Design review of the part built by this model. Coordinates are the model's own, in mm. A direction names the side the tool comes from. Coordinates: 2 decimals unless noted, no trailing zeros. Order: outer loops, then holes, each group sorted by start corner. A loop starts at its lowest first (then second) coordinate and runs counter-clockwise, first axis right, second up. Notation, with made-up numbers: M 5.25,73.25 L 12.25,73.25 A23 ccw 12.25,110.25 Z; hole C 73,24.25 d3. An arc over 180 degrees is marked long. Answer in a Markdown table with one row per item.
from build123d import *

# Parameters (mm, degrees)
SKETCH1_R           = 4.7625
BOSS_EXTRUDE1_DEPTH = 65.1002
SKETCH2_W           = 9.525
SKETCH2_H           = 2.54
CUT_EXTRUDE1_DEPTH  = 3.175
CHAMFER1_SIZE       = 0.508


with BuildPart() as part:
    # Sketch1 → Boss-Extrude1 (new body)
    with BuildSketch(Plane.XY):
        Circle(SKETCH1_R)
    extrude(amount=BOSS_EXTRUDE1_DEPTH)

    # Sketch2 → Cut-Extrude1 (cut)
    with BuildSketch(Plane.XY.offset(65.1002)):
        Rectangle(SKETCH2_W, SKETCH2_H)
    extrude(amount=-CUT_EXTRUDE1_DEPTH, mode=Mode.SUBTRACT)

    # Chamfer1
    chamfer1_edges = [part.edges().sort_by_distance(p)[0] for p in [
        (0, 4.7625, 65.1002),
        (0, -4.7625, 65.1002),
    ]]
    chamfer(chamfer1_edges, length=CHAMFER1_SIZE)


solid = part.part
(1) Insertion check: pin 1 Ø5 at (x, z) = (3, 56.5) entering from +Y; pin 2 Ø0.8 at (x, y) = (1, 0.5) entering from +Z. Each pin has a flat end and moves straight along its axis. Give the tip position at first contact, or say it passes through.
Return value:
| item | result |
|---|---|
| pin 1 | stops at y = 4.74 |
| pin 2 | stops at z = 61.93 |
(2) Draft analysis for pull direction Y (two halves, no side actions). For faces 3 (the conical face through (-0.08, -4.391, 64.963)), 4 (the flat face through (0, 0, 0)), 5 (the flat face through (0, 1.27, 64)), 6 (the conical face through (0.08, 4.391, 64.963)), state which applies: pulls with the +Y half, pulls with the -Y half, needs draft (parallel to the pull), parting line crosses it, or undercut.
Return value:
| item | result |
|---|---|
| face 3 | pulls with the -Y half |
| face 4 | needs draft |
| face 5 | undercut |
| face 6 | pulls with the +Y half |
(3) For line 1 along X through (y, z) = (-2.5, 52.5); line 2 along Z through (x, y) = (-2.75, -1); line 3 along X through (y, z) = (1.25, 17.5), list the stretches that pass through material, from the lowest coordinate up. Write a range as from..to.
Return value:
| item | result |
|---|---|
| line 1 | x = -4.05..4.05 |
| line 2 | z = 0..61.93 |
| line 3 | x = -4.6..4.6 |
(4) Add section A-A, the plane y = 0. Give the boundary of the cut face in (x, z).
Return value:
| item | result |
|---|---|
| outline | M -4.76,0 L 4.76,0 L 4.76,61.93 L -4.76,61.93 Z |
(5) For faces 1 (the flat face through (0, 2, 65.1)), 2 (the flat face through (0, -1.27, 64)), list the 3-axis set-ups (+Z, -Z, +X, -X, +Y, -Y) from which the entire face can be reached by the end or side of a thin tool; tool diameter is ignored.
Return value:
| item | result |
|---|---|
| face 1 | +Z, +X, -X, +Y, -Y |
| face 2 | +Z, +X, -X |
